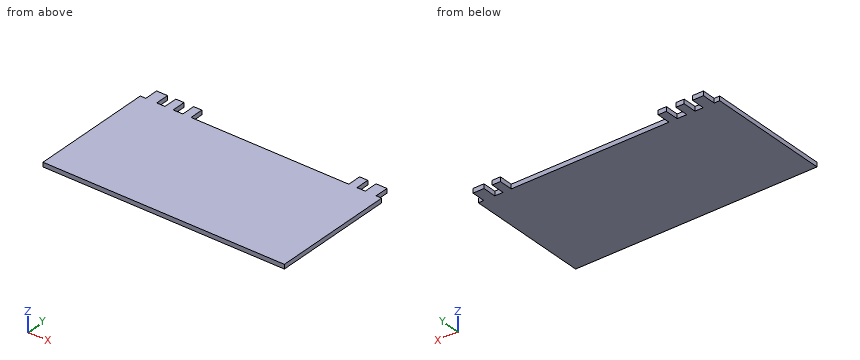
Autodesk Inventor part; units mm, degrees
ref_plane "YZ Plane" through (0, 0, 0) normal (1, 0, 0) x (0, 1, 0)
ref_plane "XZ Plane" through (0, 0, 0) normal (0, 1, 0) x (-1, 0, 0)
ref_plane "XY Plane" through (0, 0, 0) normal (0, 0, 1) x (1, 0, 0)
sketch "Sketch1" plane through (0, 0, 0) normal (0, 0, 1) x (1, 0, 0)
  line L0 (-44, -22.5) -> (44, -22.5)
  line L1 (44, -22.5) -> (44, 22.5)
  line L2 (44, 22.5) -> (-44, 22.5)
  line L3 (-44, 22.5) -> (-44, -22.5)
  line L4 (-44, -22.5) -> (44, 22.5) construction
  line L5 (44, -22.5) -> (-44, 22.5) construction
  line L6 (-42, 22.5) -> (-42, 27.5)
  line L7 (-42, 27.5) -> (-38, 27.5)
  line L8 (-38, 27.5) -> (-38, 22.5)
  line L9 (-35, 22.5) -> (-35, 27.5)
  line L10 (-35, 27.5) -> (-32, 27.5)
  line L11 (-32, 27.5) -> (-32, 22.5)
  line L12 (-28.5, 22.5) -> (-28.5, 27.5)
  line L13 (-28.5, 27.5) -> (-25.5, 27.5)
  line L14 (-25.5, 27.5) -> (-25.5, 22.5)
  line L15 (32, 22.5) -> (32, 27.5)
  line L16 (32, 27.5) -> (35, 27.5)
  line L17 (35, 27.5) -> (35, 22.5)
  line L18 (38, 22.5) -> (38, 27.5)
  line L19 (38, 27.5) -> (42, 27.5)
  line L20 (42, 27.5) -> (42, 22.5)
  point P0 (0, 0)
  point P1 (-28.5, 25)
  point P2 (-40, 27.5)
  dimension "d0" = 45
  dimension "d1" = 88
  dimension "d2" = 4
  dimension "d3" = 3
  dimension "d4" = 3
  dimension "d5" = 3
  dimension "d6" = 4
  dimension "d7" = 2
  dimension "d8" = 3
  dimension "d9" = 3.5
  dimension "d10" = 2
  dimension "d11" = 3
  dimension "d12" = 5
extrude "Extrusion1" add sketch "Sketch1" along normal blind 1.6
properties part number "PCB_2"
Verification items for the finished model (mm, model axes). Coordinates: 2 decimals unless noted, no trailing zeros. Order: outer loops, then holes, each group sorted by start corner. A loop starts at its lowest first (then second) coordinate and runs counter-clockwise, first axis right, second up. Notation, with made-up numbers: M 82,-3.5 L 140,-3.5 A12 ccw 140,17.5 Z; hole C 82.5,65.5 d6. An arc over 180 degrees is marked long. One line per item, written item: value. Start each with the question number.
Item 1: Gauge pin test, flat ends, axial feed: pin 1 (0.5 mm diameter, centred on y = 25, z = 1, fed in from +X); pin 2 (0.5 mm diameter, centred on x = 43.5, z = 0.5, fed in from +Y). Record the tip position at first contact, or that the pin passes through.
Item 2: Sectioned sample at B-B (x = 18). Enter the section's corners in (y, z), then the cut area to 3 significant figures.
Item 3: Scan lines: probe 1 along X at (y, z) = (23.5, 0.95); probe 2 along Y at (x, z) = (-24, 1.15). Record each from-to range of solid material in increasing order.
Item 4: Sectioned sample at A-A (z = 1.25). Enter the section's corners in (x, y).
Conclusion:
1. pin 1: stops at x = 42
1. pin 2: stops at y = 22.5
2. outline: M -22.5,0 L 22.5,0 L 22.5,1.6 L -22.5,1.6 Z
2. area: 72.0 mm^2
3. probe 1: x = -42 to -38, -35 to -32, -28.5 to -25.5, 32 to 35, 38 to 42
3. probe 2: y = -22.5 to 22.5
4. outline: M -44,-22.5 L 44,-22.5 L 44,22.5 L 42,22.5 L 42,27.5 L 38,27.5 L 38,22.5 L 35,22.5 L 35,27.5 L 32,27.5 L 32,22.5 L -25.5,22.5 L -25.5,27.5 L -28.5,27.5 L -28.5,22.5 L -32,22.5 L -32,27.5 L -35,27.5 L -35,22.5 L -38,22.5 L -38,27.5 L -42,27.5 L -42,22.5 L -44,22.5 Z
